Geometry check sheet. Reference: the model listing, model coordinates, mm. Face numbers are marked on the shaded views. A direction names the side the tool comes from. Round coordinates to 2 decimals unless told otherwise and drop trailing zeros. Order: outer loops, then holes, each group sorted by start corner. A loop starts at its lowest first (then second) coordinate and runs counter-clockwise, first axis right, second up.
(1) Cross-section at A-A on y = 60.75. Enter the section's corners in (x, z).
(2) Cross-section at B-B on z = 107.75. Enter the section's corners in (x, y), and give its area (3 significant figures).
(3) Draft check along Y on the marked faces 3, 4 and 5. Enter one of: pulls with the +Y half, pulls with the -Y half, needs draft (parallel to the pull), parting line crosses it, or undercut.
(4) Set-up check for the marked faces 1 and 2: record each of +Z, -Z, +X, -X, +Y, -Y from which the full face is reachable in a straight line by a thin tool's end or side.
(5) Cross-section at C-C on x = 62.5. Enter the section's corners in (y, z).
(6) Thickness scan on L1, parallel to Z at x = 58.5, y = 60; L2, parallel to Z at x = 59.5, y = 59; L3, parallel to Y at x = 58, z = 100.75. Record the ranges inside material, lowest first.
(7) Cross-section at D-D on z = 113.25. Enter the section's corners in (x, y), and give its area (3 significant figures).
(8) Gauge pin test, flat ends, axial feed: P1, Ø1, axis at x = 61.5, y = 57.5, coming from the +Z side; P2, Ø3, axis at x = 60, y = 58, coming from the -Z side; P3, Ø1.5, axis at x = 61, z = 101, coming from the +Y side; P4, Ø3, axis at x = 62, z = 112.5, coming from the -Y side. Record the tip position at first contact, or that the pin passes through.
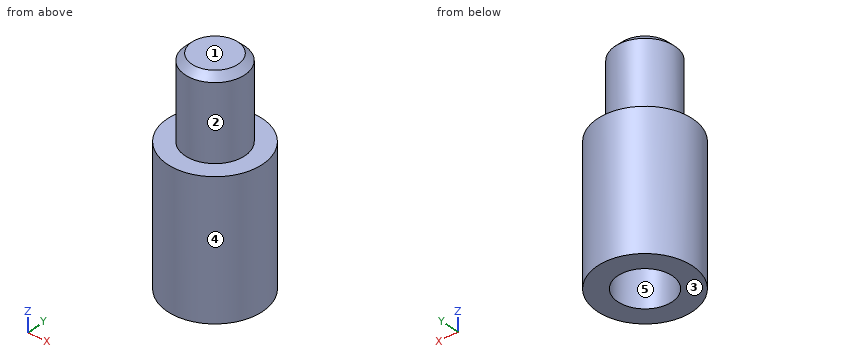
from build123d import *

# Parameters (mm, degrees)
SKETCH1_R           = 3.5
BOSS_EXTRUDE1_DEPTH = 7
SKETCH2_R           = 3.5
SKETCH2_R_2         = 2
BOSS_EXTRUDE2_DEPTH = 3
SKETCH3_R           = 2.2
BOSS_EXTRUDE3_DEPTH = 6
CHAMFER1_SIZE       = 0.5


with BuildPart() as part:
    # Sketch1 → Boss-Extrude1 (new body)
    with BuildSketch(Plane(origin=(0, 0, 107.93542322), x_dir=(-1, 0, 0), z_dir=(0, 0, -1))):
        with Locations((-59.79735108, 58.015798494)):
            Circle(SKETCH1_R)
    extrude(amount=BOSS_EXTRUDE1_DEPTH)

    # Sketch2 → Boss-Extrude2 (add)
    with BuildSketch(Plane(origin=(0, 0, 100.93542322), x_dir=(-1, 0, 0), z_dir=(0, 0, -1))):
        with Locations((-59.79735108, 58.015798494)):
            Circle(SKETCH2_R)
        with Locations((-59.79735108, 58.015798494)):
            Circle(SKETCH2_R_2, mode=Mode.SUBTRACT)
    extrude(amount=BOSS_EXTRUDE2_DEPTH)

    # Sketch3 → Boss-Extrude3 (add)
    with BuildSketch(Plane.XY.offset(107.93542322)):
        with Locations((59.79735108, 58.015798494)):
            Circle(SKETCH3_R)
    extrude(amount=BOSS_EXTRUDE3_DEPTH)

    # Chamfer1
    chamfer1_edges = [part.edges().sort_by_distance(p)[0] for p in [
        (57.59735108, 58.015798494, 113.93542322),
    ]]
    chamfer(chamfer1_edges, length=CHAMFER1_SIZE)


solid = part.part
Found:
1. outline: (57.61, 97.94) - (61.98, 97.94) - (61.98, 107.94) - (57.61, 107.94) - close
2. outline: circle Ø7 at (59.8, 58.02)
2. area: 38.5 mm2
3. face 3: needs draft
3. face 4: parting line crosses it
3. face 5: undercut
4. face 1: +Z, +X, -X, +Y, -Y
4. face 2: +Z
5. outline: (55.79, 97.94) - (60.24, 97.94) - (60.24, 107.94) - (55.79, 107.94) - close
6. L1: z = 97.94 to 107.94
6. L2: z = 100.94 to 113.94
6. L3: y = 55.01 to 57.14, 58.89 to 61.02
7. outline: circle Ø4.4 at (59.8, 58.02)
7. area: 15.2 mm2
8. P1: stops at z = 113.94
8. P2: stops at z = 100.94
8. P3: stops at y = 61.49
8. P4: stops at y = 55.93
